Geometry check sheet. Reference: the model listing, model coordinates, mm. Round coordinates to 2 decimals unless told otherwise and drop trailing zeros. Order: outer loops, then holes, each group sorted by start corner. A loop starts at its lowest first (then second) coordinate and runs counter-clockwise, first axis right, second up.
(1) Release check for a two-part mould opening along X. For faces 1 (the face through (-127, 0, 0)), 2 (the face through (-62.61, -3.17, 0.14)), 3 (the face through (-118.495, -0.044, 0.359)) record: +X half, -X half, draft (parallel to the pull), parting line (faces both ways), or undercut.
(2) Sectioned sample at B-B (x = -111). Record the boundary of the cut face in (y, z) (3 decimals), plus the area to 3 significant figures.
(3) Material ranges on line 1 along X through (y, z) = (2.5, 0); line 2 along Z through (x, y) = (-94.5, -0.5), recorded low to high.
(4) Go/stop test with flat-tipped pins: pin 1 (3 mm diameter, centred on x = -105.5, z = -2, fed in from -Y); pin 2 (1.5 mm diameter, centred on x = -41.5, y = -1, fed in from -Z); pin 3 (1 mm diameter, centred on x = -15.5, y = 1.5, fed in from +Z). Record where each tip stops, or that it passes through.
(5) Sectioned sample at A-A (y = 0). Record the boundary of the cut face in (x, z) (3 decimals), plus the area to 3 significant figures.
from build123d import *

# Parameters (mm, degrees)
F0_R     = 3.175
F1_DEPTH = 127
F4_DEPTH = 12.7
F2_R     = 1.1938
F5_DEPTH = 12.7


with BuildPart() as f1:
    # F0 (on Right) → F1 (new body)
    with BuildSketch(Plane.YZ):
        Circle(F0_R)
    extrude(amount=-F1_DEPTH)

    # F3 (on Front) → F4 (cut, symmetric)
    with BuildSketch(Plane.XZ):
        Polygon((0, -3.175), (0, -0.381), (-25.4, -3.175), align=None)
        Polygon((-25.4, 3.175), (0, 0.381), (0, 3.175), align=None)
    extrude(amount=F4_DEPTH, both=True, mode=Mode.SUBTRACT)

    # F2 (on Front) → F5 (cut, symmetric)
    with BuildSketch(Plane.XZ):
        with Locations((-119.634, 0)):
            Circle(F2_R)
    extrude(amount=F5_DEPTH, both=True, mode=Mode.SUBTRACT)


solid = f1.part
Answer below:
1. face 1: -X half
1. face 2: draft
1. face 3: undercut
2. outline: circle Ø6.35 at (0, 0)
2. area: 31.7 mm2
3. line 1: x = -127 to -120.83, -118.44 to 0
3. line 2: z = -3.14 to 3.14
4. pin 1: stops at y = -3.14
4. pin 2: stops at z = -3.17
4. pin 3: stops at z = 2.14
5. outline: (-127, -3.175) - (-25.4, -3.175) - (0, -0.381) - (0, 0.381) - (-25.4, 3.175) - (-127, 3.175) - close; hole circle Ø2.388 at (-119.634, 0)
5. area: 731 mm2
